Autodesk Inventor part; units mm, degrees
ref_plane "YZ Plane" through (0, 0, 0) normal (1, 0, 0) x (0, 1, 0)
ref_plane "XZ Plane" through (0, 0, 0) normal (0, 1, 0) x (-1, 0, 0)
ref_plane "XY Plane" through (0, 0, 0) normal (0, 0, 1) x (1, 0, 0)
sketch "Sketch1" plane through (0, 0, 0) normal (0, 0, 1) x (1, 0, 0)
  line L0 (0, 0) -> (50, 0)
  line L1 (50, 0) -> (50, 40)
  line L2 (50, 40) -> (56.731, 40)
  line L3 (56.731, 40) -> (56.731, 20)
  line L4 (56.731, 20) -> (50, 20)
  line L5 (50, 20) -> (50, 40)
  line L6 (10, 3.269) -> (30, 3.269)
  line L7 (30, 3.269) -> (30, 10)
  line L8 (30, 10) -> (10, 10)
  line L9 (10, 10) -> (10, 3.269)
  line L10 (0, 10) -> (10, 10)
  line L11 (30, 10) -> (50, 10)
  line L12 (0, 10) -> (0, 0)
  line L13 (0, 10) -> (0, 15)
  line L14 (0, 15) -> (45, 55)
  line L15 (50, 40) -> (50, 55)
  line L16 (50, 55) -> (45, 55)
  point P0 (20, 3.269)
  point P1 (20, 0)
  dimension "d2" = 20
  dimension "d3" = 20
  dimension "d5" = 6.731
  dimension "d6" = 10
  dimension "d9" = 10
  dimension "d11" = 20
  dimension "d12" = 20
  dimension "d14" = 5
  dimension "d16" = 15
  dimension "d17" = 5
extrude "Extrusion1" add sketch "Sketch1" along normal blind 6.731
fillet "Fillet1" radius 1.5875 2 edges at (45, 55, 3.3655) (0, 0, 3.3655)
sketch "Sketch3" plane through (0, 0, 6.731) normal (0, 0, 1) x (1, 0, 0)
  line L0 (45, 55) -> (0, 15)
  line L1 (3.2333, 17.874) -> (5.7738, 15.0159)
  line L2 (5.7738, 15.0159) -> (6.8292, 15.954)
  line L3 (6.8292, 15.954) -> (8.9392, 13.5803)
  line L4 (8.9392, 13.5803) -> (7.8838, 12.6422)
  line L5 (7.8838, 12.6422) -> (9.8769, 10.3999)
  line L6 (9.8769, 10.3999) -> (7.5032, 8.2899)
  line L7 (7.5032, 8.2899) -> (5.5101, 10.5322)
  line L8 (5.5101, 10.5322) -> (4.4547, 9.5941)
  line L9 (4.4547, 9.5941) -> (2.3447, 11.9678)
  line L10 (2.3447, 11.9678) -> (3.4, 12.9059)
  line L11 (3.4, 12.9059) -> (0.8595, 15.764)
  line L12 (37.8802, 48.6713) -> (40.4207, 45.8132)
  line L13 (40.4207, 45.8132) -> (39.3654, 44.8751)
  line L14 (39.3654, 44.8751) -> (41.4754, 42.5013)
  line L15 (41.4754, 42.5013) -> (42.5307, 43.4394)
  line L16 (42.5307, 43.4394) -> (44.5238, 41.1972)
  line L17 (44.5238, 41.1972) -> (46.8976, 43.3072)
  line L18 (46.8976, 43.3072) -> (44.9045, 45.5494)
  line L19 (44.9045, 45.5494) -> (45.9598, 46.4875)
  line L20 (45.9598, 46.4875) -> (43.8498, 48.8613)
  line L21 (43.8498, 48.8613) -> (42.7945, 47.9232)
  line L22 (42.7945, 47.9232) -> (40.254, 50.7813)
  dimension "d24" = 3.176
  dimension "d25" = 10
  dimension "d26" = 3
  dimension "d27" = 6
  dimension "d28" = 1.15
  dimension "d29" = 6.35
extrude "Extrusion3" cut sketch "Sketch3" against normal up to next
equation "\"d5\" = THICKB"
equation "\"d7\" = THICKB"
equation "\"THICKA\" = 3.175"
equation "\"THICKB\" = 6.731"
equation "\"THICKC\" = 12.7"
equation "\"THICKPLY\" = 5"
equation "\"MAGDIA\" = 9.5"
equation "\"BALLDIA\" = 12"
properties part number "Mount_LCD_End"
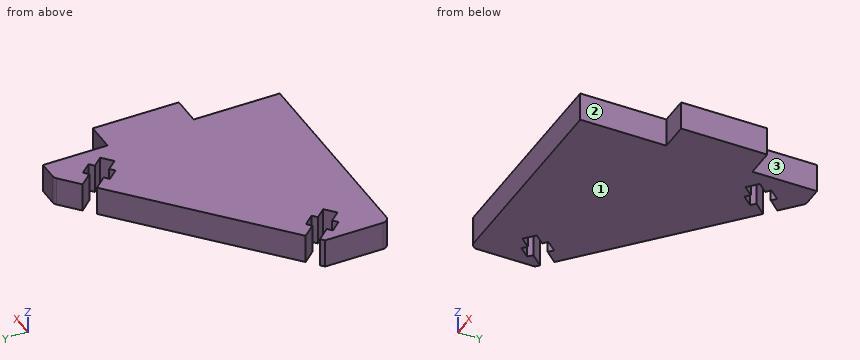
Geometry: final body of the model. Coordinates: model frame, mm. Face numbers are marked on the shaded views. A direction names the side the tool comes from. Coordinates: 2 decimals unless noted, no trailing zeros. Order: outer loops, then holes, each group sorted by start corner. A loop starts at its lowest first (then second) coordinate and runs counter-clockwise, first axis right, second up. Notation, with made-up numbers: M 49.25,63.5 L 96.25,63.5 A26 ccw 96.25,92.5 Z; hole C -38,17 d5. An arc over 180 degrees is marked long. Answer as CSV lines item,"result".
Q1. Section B-B on y = 5. Return the cut outline in (x, z).
Answers:
outline,"M 0,0 L 50,0 L 50,6.73 L 0,6.73 Z"
Q2. Set-up query: the marked faces 1, 2 and 3. Return all of +Z, -Z, +X, -X, +Y, -Y with unobstructed straight access to the full face (end or side cutting, diameter ignored); none if empty.
Answers:
face 1,"-Z, +X, -X, +Y, -Y"
face 2,"+Z, -Z, +X, -Y"
face 3,"+Z, -Z, +X, +Y"
Q3. Section A-A on x = 52. Return the cut outline in (y, z).
Answers:
outline,"M 20,0 L 40,0 L 40,6.73 L 20,6.73 Z"
Q4. First-contact query: P1, Ø2, axis at y = 7.5, z = 4.5, coming from the +X side; P2, Ø2, axis at x = 54, z = 3, coming from the +Y side; P3, Ø2, axis at y = 16.5, z = 1.5, coming from the -X side. Flat tips, straight axial feed; report the tip coordinate or a pass-through.
Answers:
P1,"stops at x = 50"
P2,"stops at y = 40"
P3,"stops at x = 0.56"
Q5. Line query: probe 1 along Y at (x, z) = (52, 2.75); probe 2 along Y at (x, z) = (42.5, 2.5); probe 3 along X at (y, z) = (45.5, 2.25). Output: solid intervals per line, ascending. Write a range as [from, to].
Answers:
probe 1,"y = [20, 40]"
probe 2,"y = [0, 43.41], [48.25, 52.78]"
probe 3,"x = [34.31, 40.07], [44.95, 50]"
